from build123d import *

# Parameters (mm, degrees)
F0_W      = 121
F0_H      = 99
F0_W_2    = 117
F0_H_2    = 95
F1_DEPTH  = 15
F2_W      = 121
F2_H      = 99
F3_DEPTH  = 28
F4_R      = 2
F5_DEPTH  = 8
F6_W      = 6
F6_H      = 3
F6_W_2    = 5
F7_DEPTH  = 80
F8_W      = 71
F8_H      = 6
F9_DEPTH  = 1
F10_W     = 30
F10_H     = 65
F11_DEPTH = 25
F12_R     = 2
F13_R     = 1.5
F14_DEPTH = 4.5


with BuildPart() as f1:
    # F0 (on Top) → F1 (new body)
    with BuildSketch(Plane.XY):
        Rectangle(F0_W, F0_H)
        Rectangle(F0_W_2, F0_H_2, mode=Mode.SUBTRACT)
    extrude(amount=-F1_DEPTH)

    # F2 (on face) → F3 (join)
    with BuildSketch(Plane.XY):
        Rectangle(F2_W, F2_H)
        Polygon((-35, 40), (26, 40), (26, -40), (-35, -40), (-45, -40), (-45, 40), align=None, mode=Mode.SUBTRACT)
    extrude(amount=F3_DEPTH)

    # F4 (on face) → F5 (cut)
    with BuildSketch(Plane(origin=(0, 0, 0), x_dir=(1, 0, 0), z_dir=(0, 0, -1))):
        with Locations((-54, 35.5)):
            Circle(F4_R)
        with Locations((-54, -41.5)):
            Circle(F4_R)
        with Locations((36.5, 35.5)):
            Circle(F4_R)
        with Locations((36.5, -41.5)):
            Circle(F4_R)
    extrude(amount=-F5_DEPTH, mode=Mode.SUBTRACT)

    # F6 (on face) → F7 (join, through all)
    with BuildSketch(Plane(origin=(0, -40, 0), x_dir=(-1, 0, 0), z_dir=(0, 1, 0))):
        with Locations((42, 26.5)):
            Rectangle(F6_W, F6_H)
        with Locations((31.5, 26.5)):
            Rectangle(F6_W_2, F6_H)
        with Locations((21.5, 26.5)):
            Rectangle(F6_W_2, F6_H)
        with Locations((11.5, 26.5)):
            Rectangle(F6_W_2, F6_H)
        with Locations((1.5, 26.5)):
            Rectangle(F6_W_2, F6_H)
        with Locations((-8.5, 26.5)):
            Rectangle(F6_W_2, F6_H)
        with Locations((-18.5, 26.5)):
            Rectangle(F6_W_2, F6_H)
    extrude(amount=F7_DEPTH)

    # F8 (on face) → F9 (cut)
    with BuildSketch(Plane(origin=(0, 0, 0), x_dir=(1, 0, 0), z_dir=(0, 0, -1))):
        with Locations((-9.5, 43)):
            Rectangle(F8_W, F8_H)
        with Locations((-9.5, -43)):
            Rectangle(F8_W, F8_H)
    extrude(amount=-F9_DEPTH, mode=Mode.SUBTRACT)

    # F10 (on face) → F11 (cut)
    with BuildSketch(Plane(origin=(0, 0, 0), x_dir=(1, 0, 0), z_dir=(0, 0, -1))):
        with Locations((41, -2.5)):
            Rectangle(F10_W, F10_H)
    extrude(amount=-F11_DEPTH, mode=Mode.SUBTRACT)

    # F12
    f12_edges = [f1.edges().sort_by_distance(p)[0] for p in [
        (-60.5, 49.5, 6.5),
        (-60.5, 0, 28),
        (0, 49.5, 28),
        (-60.5, -49.5, 6.5),
        (0, -49.5, 28),
        (60.5, -49.5, 6.5),
        (60.5, 0, 28),
        (60.5, 49.5, 6.5),
    ]]
    fillet(f12_edges, radius=F12_R)

    # F13 (on face) → F14 (cut, through all)
    with BuildSketch(Plane.YZ.offset(60.5)):
        with Locations((0, 5)):
            Circle(F13_R)
    extrude(amount=-F14_DEPTH, mode=Mode.SUBTRACT)


solid = f1.part
The model under review builds one solid part; all positions refer to its coordinate system, in mm. A direction names the side the tool comes from. Coordinates: 2 decimals unless noted, no trailing zeros. Loops run counter-clockwise (first coordinate to the right, second up) from the corner with the lowest first, then second, coordinate; pieces in that order, holes last.
(1) Wall thickness on L1, parallel to Y at x = -54, z = 3; L2, parallel to X at y = 41.5, z = 5.5; L3, parallel to Y at x = 36.5, z = 5.25: over which ranges is each line inside the solid? List them lowest first.
Determined:
L1: y = -49.5 to -37.5, -33.5 to 39.5, 43.5 to 49.5
L2: x = -60.5 to -56, -52 to 34.5, 38.5 to 60.5
L3: y = -49.5 to -37.5, -33.5 to -30, 35 to 39.5, 43.5 to 49.5
(2) Consider section B-B, the plane z = 19.5. Give the boundary of the cut face in (x, y).
Determined:
outline: (-60.5, -47.5) arc R2 ccw to (-58.5, -49.5) - (58.5, -49.5) arc R2 ccw to (60.5, -47.5) - (60.5, 47.5) arc R2 ccw to (58.5, 49.5) - (-58.5, 49.5) arc R2 ccw to (-60.5, 47.5) - close; hole (-45, -40) - (26, -40) - (26, -30) - (56, -30) - (56, 35) - (26, 35) - (26, 40) - (-45, 40) - close
(3) Insertion check: P1, Ø6, axis at x = -17.5, y = 30.5, coming from the -Z side; P2, Ø2.5, axis at y = 0, z = 5, coming from the +X side; P3, Ø5, axis at x = -20, y = -42.5, coming from the -Z side. Each pin has a flat end and moves straight along its axis. Give the tip position at first contact, or say it passes through.
Determined:
P1: stops at z = 25
P2: stops at x = -45
P3: stops at z = 1
(4) Tool access review of faces 3 (the flat face through (-42, -1, 25)), 4 (the flat face through (1, -1, 26)): name each direction out of +Z, -Z, +X, -X, +Y, -Y from which nothing blocks a thin tool from reaching the whole face with its end or side.
Determined:
face 3: -Z
face 4: +Z, -Z
(5) Draft analysis for pull direction Y (two halves, no side actions). For faces 1 (the flat face through (-1, -49.5, 5)), 2 (the flat face through (-11, -1, 25)), state which applies: +Y half, -Y half, draft (parallel to the pull), parting line (faces both ways), or undercut.
Determined:
face 1: -Y half
face 2: undercut
(6) Consider section C-C, the plane x = 36.5. Give the boundary of the cut face in (y, z).
Determined:
outline: (-49.5, -15) - (-47.5, -15) - (-47.5, 0) - (-37.5, 0) - (-37.5, 8) - (-33.5, 8) - (-33.5, 0) - (-30, 0) - (-30, 25) - (35, 25) - (35, 0) - (39.5, 0) - (39.5, 8) - (43.5, 8) - (43.5, 0) - (47.5, 0) - (47.5, -15) - (49.5, -15) - (49.5, 26) arc R2 ccw to (47.5, 28) - (-47.5, 28) arc R2 ccw to (-49.5, 26) - close
(7) Consider section A-A, the plane x = -26.5. Give the boundary of the cut face in (y, z), plus the area to 3 significant figures.
Determined:
outline: (-49.5, -15) - (-47.5, -15) - (-47.5, 0) - (-46, 0) - (-46, 1) - (-40, 1) - (-40, 28) - (-47.5, 28) arc R2 ccw to (-49.5, 26) - close; (40, 1) - (46, 1) - (46, 0) - (47.5, 0) - (47.5, -15) - (49.5, -15) - (49.5, 26) arc R2 ccw to (47.5, 28) - (40, 28) - close
area: 578 mm2
(8) Consider section D-D, the plane y = -35.5. Give the number of separate pieces and of enclosed holes in the cut face, plus the area to 3 significant figures.
Determined:
separate pieces: 8
enclosed holes: 0
area: 1,500 mm2
